CAD build for the part. Positions are in the model's coordinates, mm. A direction names the side the tool comes from. Coordinates: 2 decimals unless noted, no trailing zeros. Order: outer loops, then holes, each group sorted by start corner. A loop starts at its lowest first (then second) coordinate and runs counter-clockwise, first axis right, second up. Notation, with made-up numbers: (86, 47) - (141, 47) arc R17 cw to (141, 66) - close; hole circle Ø10 at (-33.5, 1). An arc over 180 degrees is marked (long way). Return JSON: item names as keys, results as strings.
from build123d import *

# Parameters (mm, degrees)
BOSS_EXTRUDE1_DEPTH = 6.5
FILLET4_START       = -8
FILLET4_DEPTH       = 16
FILLET4_START_2     = -34.5
FILLET4_2_DEPTH     = 69
SKETCH4_W           = 251.095983112
SKETCH4_H           = 149.113377468
CUT_EXTRUDE2_DEPTH  = 1.5
SKETCH6_R           = 6.5
BOSS_EXTRUDE3_DEPTH = 27
FILLET3_R           = 3
CUT_EXTRUDE3_DEPTH  = 18
MIRROR1_START       = 6.5
MIRROR1_OUTLINE_R   = 6.5
MIRROR1_DEPTH       = 27
MIRROR1_2_DEPTH     = 9
CUT_EXTRUDE6_REACH  = 125.858


with BuildPart() as part:
    # Sketch1 → Boss-Extrude1 (new body)
    with BuildSketch(Plane.XY):
        with BuildLine():
            Line((34.5, -13), (34.5, -67.2))
            Line((34.5, -67.2), (-34.5, -67.2))
            Line((-34.5, -67.2), (-34.5, -13))
            ThreePointArc((-34.5, -13), (-35.964466094, -9.464466094), (-39.5, -8))
            Line((-39.5, -8), (-97, -8))
            Line((-97, -8), (-97, 8))
            Line((-97, 8), (-39.5, 8))
            ThreePointArc((-39.5, 8), (-35.964466094, 9.464466094), (-34.5, 13))
            Line((-34.5, 13), (-34.5, 67.2))
            Line((-34.5, 67.2), (34.5, 67.2))
            Line((34.5, 67.2), (34.5, 13))
            ThreePointArc((34.5, 13), (35.964466094, 9.464466094), (39.5, 8))
            Line((39.5, 8), (83.5, 8))
            Line((83.5, 8), (99, 8))
            Line((99, 8), (99, -8))
            Line((99, -8), (39.5, -8))
            ThreePointArc((39.5, -8), (35.964466094, -9.464466094), (34.5, -13))
        make_face()
    extrude(amount=BOSS_EXTRUDE1_DEPTH)

    # Fillet4: read off the stored shape, not the designer's step
    # Fillet4 outline → Fillet4 (cut)
    with BuildSketch(Plane(origin=(0, 0, 0), x_dir=(1, 0, 0), z_dir=(0, 1, 0)).offset(FILLET4_START)):
        with BuildLine():
            add(Edge.make_bspline(
                [(-97, -6.5), (-94.571389667, 0), (-87.632503002, 0)],
                knots=[0, 0, 0, 1, 1, 1], degree=2, weights=[1, 0.176470588, 1]))
            Line((-87.632503002, 0), (-97, 0))
            Line((-97, 0), (-97, -6.5))
        make_face()
        with BuildLine():
            add(Edge.make_bspline(
                [(99, -6.5), (96.571389667, 0), (89.632503002, 0)],
                knots=[0, 0, 0, 1, 1, 1], degree=2, weights=[1, 0.176470588, 1]))
            Line((99, -6.5), (99, 0))
            Line((99, 0), (89.632503002, 0))
        make_face()
    extrude(amount=FILLET4_DEPTH, mode=Mode.SUBTRACT)

    # Fillet4 2 outline → Fillet4 2 (cut)
    with BuildSketch(Plane.YZ.offset(FILLET4_START_2)):
        with BuildLine():
            Line((67.2, 0), (67.2, 6.5))
            add(Edge.make_bspline(
                [(67.2, 6.5), (64.771389667, 0), (57.832503002, 0)],
                knots=[0, 0, 0, 1, 1, 1], degree=2, weights=[1, 0.176470588, 1]))
            Line((57.832503002, 0), (67.2, 0))
        make_face()
        with BuildLine():
            Line((-67.2, 0), (-57.832503002, 0))
            add(Edge.make_bspline(
                [(-67.2, 6.5), (-64.771389667, 0), (-57.832503002, 0)],
                knots=[0, 0, 0, 1, 1, 1], degree=2, weights=[1, 0.176470588, 1]))
            Line((-67.2, 6.5), (-67.2, 0))
        make_face()
    extrude(amount=FILLET4_2_DEPTH, mode=Mode.SUBTRACT)

    # Sketch4 → Cut-Extrude2 (cut)
    with BuildSketch(Plane.XY):
        Rectangle(SKETCH4_W, SKETCH4_H)
    extrude(amount=CUT_EXTRUDE2_DEPTH, mode=Mode.SUBTRACT)

    # Sketch6 → Boss-Extrude3 (add)
    with BuildSketch(Plane.XY.offset(6.5)):
        with Locations((-24.5, 29)):
            Circle(SKETCH6_R)
    extrude(amount=BOSS_EXTRUDE3_DEPTH)

    # Fillet3
    fillet3_edges = [part.edges().sort_by_distance(p)[0] for p in [
        (-31, 29, 6.5),
    ]]
    fillet(fillet3_edges, radius=FILLET3_R)

    # Sketch7 → Cut-Extrude3 (cut)
    with BuildSketch(Plane.XY.offset(33.5)):
        Polygon((-27.444486373, 29), (-25.972243186, 26.45), (-23.027756814, 26.45), (-21.555513627, 29), (-23.027756814, 31.55), (-25.972243186, 31.55), align=None)
    extrude(amount=-CUT_EXTRUDE3_DEPTH, mode=Mode.SUBTRACT)

    # Mirror1: read off the stored shape, not the designer's step
    # Mirror1 outline → Mirror1 (add)
    # profile 1 of 3: a face of its own
    with BuildSketch(Plane.XY.offset(MIRROR1_START)):
        with Locations((24.5, 29)):
            Circle(MIRROR1_OUTLINE_R)
        Polygon((21.555513627, 29), (23.027756814, 31.55), (25.972243186, 31.55), (27.444486373, 29), (25.972243186, 26.45), (23.027756814, 26.45), align=None, mode=Mode.SUBTRACT)
    # profile 2 of 3: a face of its own
    with BuildSketch(Plane.XY.offset(MIRROR1_START)):
        with Locations((-24.5, -29)):
            Circle(MIRROR1_OUTLINE_R)
        Polygon((-23.027756814, -31.55), (-25.972243186, -31.55), (-27.444486373, -29), (-25.972243186, -26.45), (-23.027756814, -26.45), (-21.555513627, -29), align=None, mode=Mode.SUBTRACT)
    # profile 3 of 3: a face of its own
    with BuildSketch(Plane.XY.offset(MIRROR1_START)):
        with Locations((24.5, -29)):
            Circle(MIRROR1_OUTLINE_R)
        Polygon((23.027756814, -26.45), (25.972243186, -26.45), (27.444486373, -29), (25.972243186, -31.55), (23.027756814, -31.55), (21.555513627, -29), align=None, mode=Mode.SUBTRACT)
    extrude(amount=MIRROR1_DEPTH)

    # Mirror1 2 outline → Mirror1 2 (add)
    with BuildSketch(Plane.XY.offset(MIRROR1_START)):
        Polygon((25.972243186, 31.55), (23.027756814, 31.55), (21.555513627, 29), (23.027756814, 26.45), (25.972243186, 26.45), (27.444486373, 29), align=None)
        Polygon((-27.444486373, -29), (-25.972243186, -31.55), (-23.027756814, -31.55), (-21.555513627, -29), (-23.027756814, -26.45), (-25.972243186, -26.45), align=None)
        Polygon((27.444486373, -29), (25.972243186, -26.45), (23.027756814, -26.45), (21.555513627, -29), (23.027756814, -31.55), (25.972243186, -31.55), align=None)
    extrude(amount=MIRROR1_2_DEPTH)

    # Mirror1 3 outline → Mirror1 3 (revolve)
    with BuildSketch(Plane(origin=(24.5, 29, 0), x_dir=(1, 0, 0), z_dir=(0, -1, 0))):
        with BuildLine():
            ThreePointArc((9.5, 6.5), (7.378679656, 7.378679656), (6.5, 9.5))
            Line((6.5, 9.5), (6.5, 6.5))
            Line((6.5, 6.5), (9.5, 6.5))
        make_face()
    revolve(axis=Axis((24.5, 29, 0), (0, 0, 1)))

    # Mirror1 4 outline → Mirror1 4 (revolve)
    with BuildSketch(Plane(origin=(-24.5, -29, 0), x_dir=(1, 0, 0), z_dir=(0, -1, 0))):
        with BuildLine():
            ThreePointArc((9.5, 6.5), (7.378679656, 7.378679656), (6.5, 9.5))
            Line((6.5, 9.5), (6.5, 6.5))
            Line((6.5, 6.5), (9.5, 6.5))
        make_face()
    revolve(axis=Axis((-24.5, -29, 0), (0, 0, 1)))

    # Mirror1 5 outline → Mirror1 5 (revolve)
    with BuildSketch(Plane(origin=(24.5, -29, 0), x_dir=(1, 0, 0), z_dir=(0, -1, 0))):
        with BuildLine():
            ThreePointArc((9.5, 6.5), (7.378679656, 7.378679656), (6.5, 9.5))
            Line((6.5, 9.5), (6.5, 6.5))
            Line((6.5, 6.5), (9.5, 6.5))
        make_face()
    revolve(axis=Axis((24.5, -29, 0), (0, 0, 1)))

    # Sketch13 → Cut-Extrude6 (cut, up to next)
    with BuildSketch(Plane(origin=(0, 0, 1.5), x_dir=(-1, 0, 0), z_dir=(0, 0, -1)), mode=Mode.PRIVATE) as cut_extrude6_sk1:
        with BuildLine():
            Line((-13.5, 54.6), (-13.5, 24))
            ThreePointArc((-13.5, 24), (-14.964466094, 20.464466094), (-18.5, 19))
            Line((-18.5, 19), (-20, 19))
            ThreePointArc((-20, 19), (-23.535533906, 17.535533906), (-25, 14))
            Line((-25, 14), (-25, -14))
            ThreePointArc((-25, -14), (-23.535533906, -17.535533906), (-20, -19))
            Line((-20, -19), (-18.5, -19))
            ThreePointArc((-18.5, -19), (-14.964466094, -20.464466094), (-13.5, -24))
            Line((-13.5, -24), (-13.5, -54.6))
            ThreePointArc((-13.5, -54.6), (-12.035533906, -58.135533906), (-8.5, -59.6))
            Line((-8.5, -59.6), (8.5, -59.6))
            ThreePointArc((8.5, -59.6), (12.035533906, -58.135533906), (13.5, -54.6))
            Line((13.5, -54.6), (13.5, -24))
            ThreePointArc((13.5, -24), (14.964466094, -20.464466094), (18.5, -19))
            Line((18.5, -19), (20, -19))
            ThreePointArc((20, -19), (23.535533906, -17.535533906), (25, -14))
            Line((25, -14), (25, 14))
            ThreePointArc((25, 14), (23.535533906, 17.535533906), (20, 19))
            Line((20, 19), (18.5, 19))
            ThreePointArc((18.5, 19), (14.964466094, 20.464466094), (13.5, 24))
            Line((13.5, 24), (13.5, 54.6))
            ThreePointArc((13.5, 54.6), (12.035533906, 58.135533906), (8.5, 59.6))
            Line((8.5, 59.6), (-8.5, 59.6))
            ThreePointArc((-8.5, 59.6), (-12.035533906, 58.135533906), (-13.5, 54.6))
        make_face()
    cut_extrude6_tool1 = extrude(cut_extrude6_sk1.sketch, amount=-CUT_EXTRUDE6_REACH, mode=Mode.PRIVATE) & part.part
    add(cut_extrude6_tool1.solids().sort_by_distance((0, 0, 1.5))[0], mode=Mode.SUBTRACT)


solid = part.part
Item 1: Band-saw the part on C-C, the plane x = 58.5. List the corners of the cut face in (y, z).
Findings below:
{"outline": "(-8, 1.5) - (8, 1.5) - (8, 6.5) - (-8, 6.5) - close"}
Item 2: Mould opens along Y. For faces 1 (the flat face through (-68, -8, 4)), 2 (the flat face through (24, 26, 33.5)), 3 (the cylindrical face through (-12.07, 58.1, 3.96)) say: released by +Y, released by -Y, zero draft, split by the parting line, or undercut.
Findings below:
{"face 1": "released by -Y", "face 2": "zero draft", "face 3": "undercut"}
Item 3: Wall check: L1, parallel to Y at x = 25.5, z = 31.5; L2, parallel to X at y = -29.5, z = 11.5; L3, parallel to Y at x = -39, z = 6. Give the ranges that are in metal, low to high. Write a range as [from, to].
Findings below:
{"L1": "y = [-35.42, -31.55], [-26.45, -22.58], [22.58, 26.45], [31.55, 35.42]", "L2": "x = [-30.98, -18.02], [18.02, 30.98]", "L3": "y = [-8.03, 8.03]"}
Item 4: Drop flat-ended pins along their axis: P1, Ø4, axis at y = -41.5, z = 3, coming from the +X side; P2, Ø3, axis at x = -32, z = 22, coming from the -Y side; P3, Ø1.2, axis at x = 19, z = 3, coming from the -Y side. Give the stop position or say it passes through.
Findings below:
{"P1": "stops at x = 34.5", "P2": "stops at y = -31.5", "P3": "stops at y = -64.02"}
Item 5: Band-saw the part on A-A, the plane y = -44. List the corners of the cut face in (x, z).
Findings below:
{"outline": "(-34.5, 1.5) - (-13.5, 1.5) - (-13.5, 6.5) - (-34.5, 6.5) - close; (13.5, 1.5) - (34.5, 1.5) - (34.5, 6.5) - (13.5, 6.5) - close"}
Item 6: Band-saw the part on B-B, the plane z = 12.5. List the corners of the cut face in (x, y).
Findings below:
{"outline": "circle Ø13 at (-24.5, -29); circle Ø13 at (-24.5, 29); circle Ø13 at (24.5, -29); circle Ø13 at (24.5, 29)"}
Item 7: Which spindle directions (+Z, -Z, +X, -X, +Y, -Y) get a long thin tool onto all of the face, cutting with end or side? Do faces 4 (the flat face through (-34.5, 40, 4)), 5 (the cylindrical face through (-12, -58.17, 3.96)), 6 (the flat face through (-25, -32, 33.5)), 7 (the cylindrical face through (35.93, 9.5, 3.96)), 8 (the cylindrical face through (19.709, -24.607, 21.332)). Say none if no direction does.
Findings below:
{"face 4": "+Z, -Z, -X, +Y", "face 5": "+Z, -Z", "face 6": "+Z, +X, -X, +Y, -Y", "face 7": "+Z, -Z, +X, +Y", "face 8": "+Z"}
